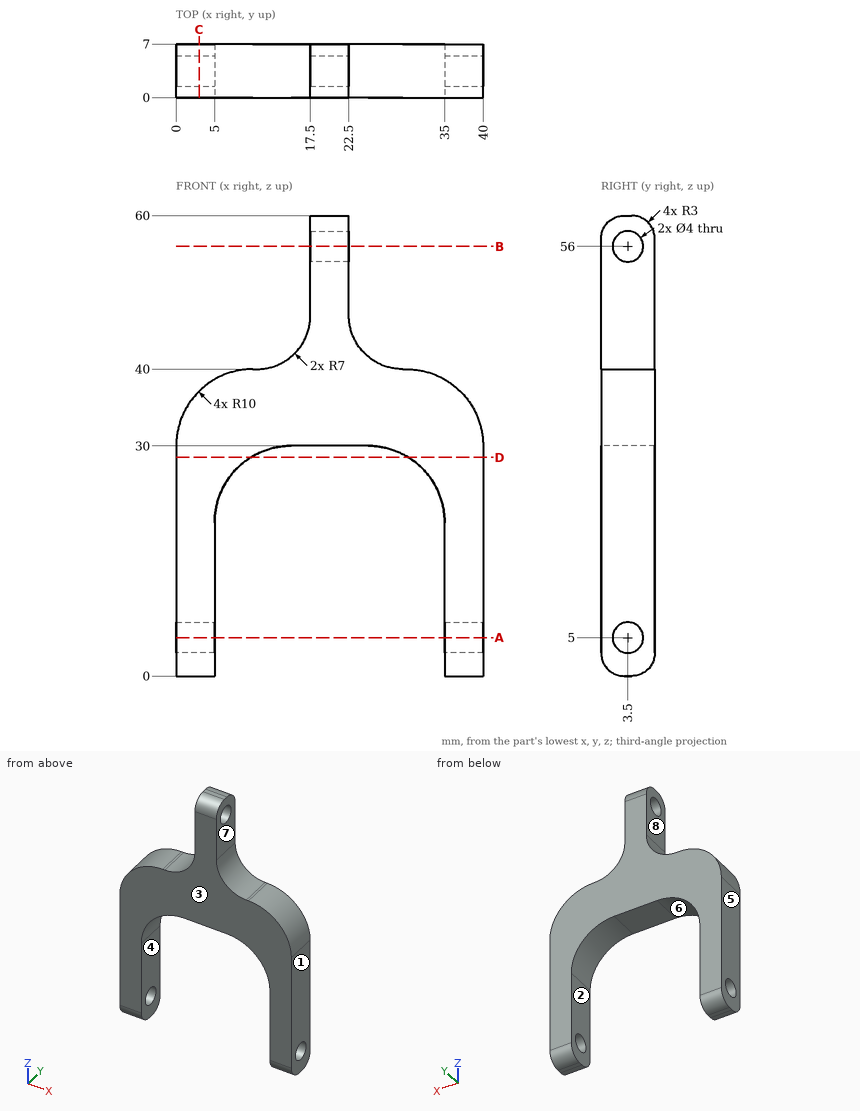
Print and shaded views of the part. All mm, measured from the part's lowest x, y and z. A direction names the side the tool comes from. Round coordinates to 2 decimals unless told otherwise and drop trailing zeros. Write each loop counter-clockwise with the first axis right and the second up, starting at its lowest first coordinate (ties: lowest second). Pieces come first, ordered by that corner, then holes. Notation, with made-up numbers: (-34.5, 38.5) - (-19.5, 38.5) arc R16 ccw to (-19.5, 58.5) - close; hole circle Ø7 at (-33, 3). An arc over 180 degrees is marked (long way). One line per item, written item: value.
(1) Cut at A-A, the plane z = 5. Give the cut face in (x, y).
Values follow:
outline: (0, 0) - (5, 0) - (5, 1.5) - (0, 1.5) - close; (0, 5.5) - (5, 5.5) - (5, 7) - (0, 7) - close; (35, 0) - (40, 0) - (40, 1.5) - (35, 1.5) - close; (35, 5.5) - (40, 5.5) - (40, 7) - (35, 7) - close
(2) Cut at B-B, the plane z = 56. Give the cut face in (x, y), plus the area to 3 significant figures.
Values follow:
outline: (17.5, 0) - (22.5, 0) - (22.5, 1.5) - (17.5, 1.5) - close; (17.5, 5.5) - (22.5, 5.5) - (22.5, 7) - (17.5, 7) - close
area: 15.0 mm²
(3) Wall check: probe 1 along Y at (x, z) = (3, 5); probe 2 along X at (y, z) = (6.5, 13); probe 3 along X at (y, z) = (4.75, 28.5). Give the ranges that are in metal, low to high.
Values follow:
probe 1: y = 0 to 1.5, 5.5 to 7
probe 2: x = 0 to 5, 35 to 40
probe 3: x = 0 to 9.73, 30.27 to 40
(4) Drop flat-ended pins along their axis: P1, Ø1.5, axis at y = 5.5, z = 51, coming from the -X side; P2, Ø2, axis at x = 19.5, y = 2.5, coming from the -Z side; P3, Ø1.5, axis at y = 1, z = 39.5, coming from the +X side. Give the stop position or say it passes through.
Values follow:
P1: stops at x = 17.5
P2: stops at z = 30
P3: stops at x = 34.84
(5) Two-plate mould, pull along X, no slides. Class the marked faces 1, 2, 3 and 4: pulls with the +X half, pulls with the -X half, needs draft (parallel to the pull), parting line crosses it, or undercut.
Values follow:
face 1: pulls with the +X half
face 2: undercut
face 3: needs draft
face 4: undercut
(6) Cut at C-C, the plane x = 3. Give the cut face in (y, z), plus the area to 3 significant figures.
Values follow:
outline: (0, 3) arc R3 ccw to (3, 0) - (4, 0) arc R3 ccw to (7, 3) - (7, 37.14) - (0, 37.14) - close; hole circle Ø4 at (3.5, 5)
area: 244 mm²
(7) 3-axis set-ups, long thin cutter, end or side, ignore diameter. For the marked faces 5, 6, 7 and 8: which of +Z, -Z, +X, -X, +Y, -Y reach the whole face in a straight line?
Values follow:
face 5: +Z, -Z, -X, +Y, -Y
face 6: -Z, +Y, -Y
face 7: +Z, +X, +Y, -Y
face 8: +Z, -X, +Y, -Y
(8) Cut at D-D, the plane z = 28.5. Give the cut face in (x, y), plus the area to 3 significant figures.
Values follow:
outline: (0, 0) - (9.73, 0) - (9.73, 7) - (0, 7) - close; (30.27, 0) - (40, 0) - (40, 7) - (30.27, 7) - close
area: 136 mm²
